Geometry: final body of the model. Coordinates: model frame, mm. Face numbers are marked on the shaded views. A direction names the side the tool comes from. Round coordinates to 2 decimals unless told otherwise and drop trailing zeros. Write each loop counter-clockwise with the first axis right and the second up, starting at its lowest first coordinate (ties: lowest second). Pieces come first, ordered by that corner, then holes. Notation, with made-up numbers: (-34.75, 67) - (-9.75, 67) arc R19 cw to (-9.75, 89) - close; hole circle Ø9 at (64.5, 10.25). An arc over 180 degrees is marked (long way). Use a Markdown table: item, result. Add a question column.
```python
from build123d import *

# Parameters (mm, degrees)
F2_R = 0.99999


# Not quite as in the source:
# - a fillet or chamfer is up to 0.001 mm smaller than in the source, because OpenCascade refuses the exact size


with BuildPart() as f1:
    # F0 (on Front) → F1 (revolve)
    with BuildSketch(Plane.XZ):
        with BuildLine():
            Line((0, 25), (0, 22))
            Line((0, 22), (3, 22))
            ThreePointArc((3, 22), (2.1213203436, 24.1213203436), (0, 25))
        make_face()
        with BuildLine():
            ThreePointArc((0, 1.5), (1.0606601718, 1.0606601718), (1.5, 0))
            Line((1.5, 0), (3.5, 0))
            Line((3.5, 0), (3.5, 3))
            Line((3.5, 3), (3, 3))
            Line((3, 3), (3, 7))
            Line((3, 7), (2, 7))
            Line((2, 7), (2, 18))
            Line((2, 18), (3, 18))
            Line((3, 18), (3, 22))
            Line((3, 22), (0, 22))
            Line((0, 22), (0, 3))
            Line((0, 3), (0, 1.5))
        make_face()
    revolve(axis=Axis((0, 0, 13.25), (0, 0, -1)))

    # F2 (radius 1 in the source; OpenCascade refuses exactly that, so slightly less here)
    f2_edges = [f1.edges().sort_by_distance(p)[0] for p in [
        (-2, 0, 18),
        (-2, 0, 7),
    ]]
    fillet(f2_edges, radius=F2_R)


solid = f1.part
```
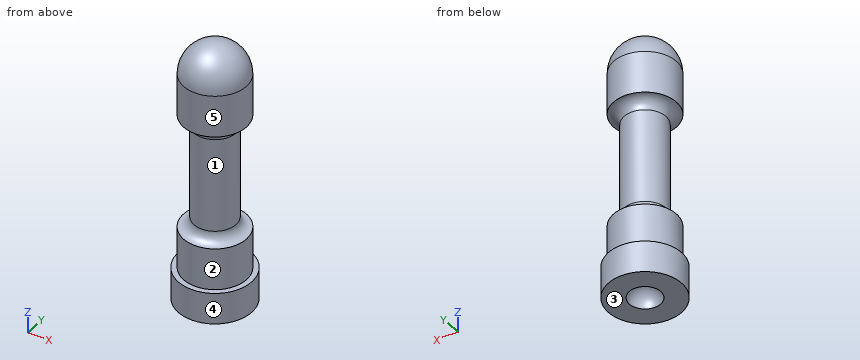
1) Section D-D, the plane x = 3.25. Return the cut outline in (y, z).
2) Set-up query: the marked faces 4 and 5. Return all of +Z, -Z, +X, -X, +Y, -Y with unobstructed straight access to the full face (end or side cutting, diameter ignored); none if empty.
3) Material intervals for L1, parallel to Z at x = 1.75, y = -3; L2, parallel to Z at x = 2.25, y = 1.25; L3, parallel to Y at x = 0, z = 20, sorted ascending. Write a range as from..to.
4) Section C-C, the plane z = 16.75. Return the cut outline in (x, y).
5) Pin query (flat end, axial travel): P1, Ø4, axis at y = 1.5, z = 21, coming from the -X side; P2, Ø2, axis at x = -2, z = 16.5, coming from the -Y side; P3, Ø1.8, axis at x = 1.5, y = 1, coming from the +Z side. Return the tip coordinate at first contact, or that it passes through.
6) Draft query along Z for the marked faces 1, 2 and 3. Return one class per face: released by +Z, released by -Z, zero draft, split by the parting line, or undercut.
7) Section B-B, the plane z = 2.5. Return the cut outline in (x, y).
Output values:
| question | item | result |
|---|---|---|
| 1 | outline | (-1.3, 0) - (1.3, 0) - (1.3, 3) - (-1.3, 3) - close |
| 2 | face 4 | +Z, -Z |
| 2 | face 5 | +Z |
| 3 | L1 | z = 0..3 |
| 3 | L2 | z = 0..7.1, 17.9..23.54 |
| 3 | L3 | y = -3..3 |
| 4 | outline | circle Ø4 at (0, 0) |
| 5 | P1 | stops at x = -3 |
| 5 | P2 | stops at y = -1.73 |
| 5 | P3 | stops at z = 24.86 |
| 6 | face 1 | undercut |
| 6 | face 2 | zero draft |
| 6 | face 3 | released by -Z |
| 7 | outline | circle Ø7 at (0, 0) |
